For this review, take the finished solid that the model builds, in its own axes (mm). Face numbers are marked on the shaded views. Round coordinates to 2 decimals unless told otherwise and drop trailing zeros. Order: outer loops, then holes, each group sorted by start corner. A loop starts at its lowest first (then second) coordinate and runs counter-clockwise, first axis right, second up.
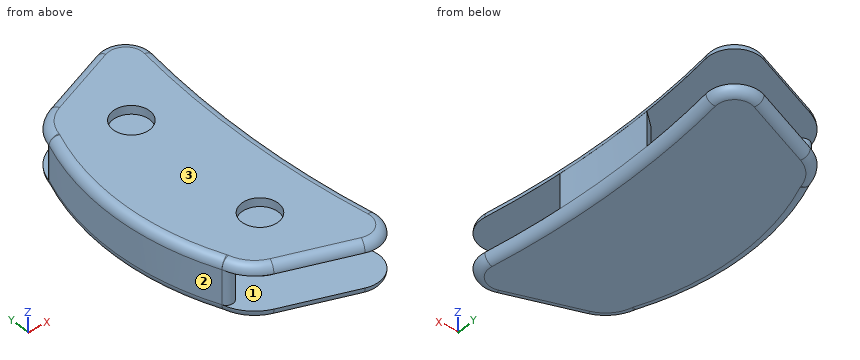
```python
from build123d import *

# Parameters (mm, degrees)
F1_DEPTH  = 2
F2_R      = 5.6
F3_DEPTH  = 1.5
F5_DEPTH  = 10
F7_DEPTH  = 2
F8_R      = 1.99999
F9_R      = 4.25
F10_DEPTH = 2


# Not quite as in the source:
# - a fillet or chamfer is up to 0.001 mm smaller than in the source, because OpenCascade refuses the exact size


with BuildPart() as f1:
    # F0 (on Top) → F1 (new body)
    with BuildSketch(Plane.XY):
        with BuildLine():
            Line((8.2361189543, 36.6168409437), (-7.9935965644, 30.5207371811))
            ThreePointArc((-7.9935965644, 30.5207371811), (-11.9662543406, 27.7862465208), (-14.1970285873, 23.510372898))
            ThreePointArc((-14.1970285873, 23.510372898), (-17, 0), (-14.1970285873, -23.510372898))
            ThreePointArc((-14.1970285873, -23.510372898), (-11.9662543406, -27.7862465208), (-7.9935965644, -30.5207371811))
            Line((-7.9935965644, -30.5207371811), (8.2361189543, -36.6168409437))
            ThreePointArc((8.2361189543, -36.6168409437), (14.1245779615, -35.6606279318), (16.2775548115, -30.0970873786))
            ThreePointArc((16.2775548115, -30.0970873786), (14, 0), (16.2775548115, 30.0970873786))
            ThreePointArc((16.2775548115, 30.0970873786), (14.1245779615, 35.6606279318), (8.2361189543, 36.6168409437))
        make_face()
    extrude(amount=F1_DEPTH)

    # F2 (on face) → F3 (cut)
    with BuildSketch(Plane.XY.offset(2)):
        with Locations((0, 17.5)):
            Circle(F2_R)
        with Locations((0, -17.5)):
            Circle(F2_R)
    extrude(amount=-F3_DEPTH, mode=Mode.SUBTRACT)

    # F4 (on Top) → F5 (join)
    with BuildSketch(Plane.XY):
        with BuildLine():
            Line((-11, -22.8789469535), (-11, 22.8789469535))
            ThreePointArc((-11, 22.8789469535), (-12.3390571638, 24.5083402847), (-14.1970285873, 23.510372898))
            ThreePointArc((-14.1970285873, 23.510372898), (-18.8404213522, 0), (-14.1970285873, -23.510372898))
            ThreePointArc((-14.1970285873, -23.510372898), (-12.3390571638, -24.5083402847), (-11, -22.8789469535))
        make_face()
        with BuildLine():
            Line((14.3490034732, 11.8101475791), (11, 9))
            Line((11, 9), (11, -9))
            Line((11, -9), (14.3490034732, -11.8101475791))
            ThreePointArc((14.3490034732, -11.8101475791), (14, 0), (14.3490034732, 11.8101475791))
        make_face()
    extrude(amount=F5_DEPTH)

    # F6 (on face) → F7 (join)
    with BuildSketch(Plane.XY.offset(10)):
        with BuildLine():
            Line((8.2361189543, 36.6168409437), (-7.9935965644, 30.5207371811))
            ThreePointArc((-7.9935965644, 30.5207371811), (-11.9662543406, 27.7862465208), (-14.1970285873, 23.510372898))
            ThreePointArc((-14.1970285873, 23.510372898), (-12.3390571638, 24.5083402847), (-11, 22.8789469535))
            Line((-11, 22.8789469535), (-11, -22.8789469535))
            ThreePointArc((-11, -22.8789469535), (-12.3390571638, -24.5083402847), (-14.1970285873, -23.510372898))
            ThreePointArc((-14.1970285873, -23.510372898), (-11.9662543406, -27.7862465208), (-7.9935965644, -30.5207371811))
            Line((-7.9935965644, -30.5207371811), (8.2361189543, -36.6168409437))
            ThreePointArc((8.2361189543, -36.6168409437), (14.1245779615, -35.6606279318), (16.2775548115, -30.0970873786))
            ThreePointArc((16.2775548115, -30.0970873786), (14, 0), (16.2775548115, 30.0970873786))
            ThreePointArc((16.2775548115, 30.0970873786), (14.1245779615, 35.6606279318), (8.2361189543, 36.6168409437))
        make_face()
        with BuildLine():
            ThreePointArc((-11, 22.8789469535), (-12.3390571638, 24.5083402847), (-14.1970285873, 23.510372898))
            ThreePointArc((-14.1970285873, 23.510372898), (-18.8404213522, 0), (-14.1970285873, -23.510372898))
            ThreePointArc((-14.1970285873, -23.510372898), (-12.3390571638, -24.5083402847), (-11, -22.8789469535))
            Line((-11, -22.8789469535), (-11, 22.8789469535))
        make_face()
    extrude(amount=F7_DEPTH)

    # F8 (radius 2 in the source; OpenCascade refuses exactly that, so slightly less here)
    f8_edges = [f1.edges().sort_by_distance(p)[0] for p in [
        (14.124578, 35.660628, 12),
        (0.121261, 33.568789, 12),
        (-11.966254, 27.786247, 12),
        (-18.840421, 0, 12),
        (-11.966254, -27.786247, 12),
        (0.121261, -33.568789, 12),
        (14.124578, -35.660628, 12),
        (14, 0, 12),
        (-18.840421, 0, 0),
        (14, 0, 0),
    ]]
    fillet(f8_edges, radius=F8_R)

    # F9 (on face) → F10 (cut)
    with BuildSketch(Plane(origin=(0, 0, 10), x_dir=(1, 0, 0), z_dir=(0, 0, -1))):
        with Locations((0, 17.5)):
            Circle(F9_R)
        with Locations((0, -17.5)):
            Circle(F9_R)
    extrude(amount=-F10_DEPTH, mode=Mode.SUBTRACT)


solid = f1.part
```
Q1. Mouldability with a two-part tool opening along Z and no side actions: class the marked faces 1, 2 and 3 as +Z half, -Z half, draft (parallel to the pull), parting line (faces both ways), or undercut.
Q2. Wall thickness on line 1 (Z direction, x = 12.5, y = 20.5); line 2 (Y direction, x = 0, z = 11); line 3 (X direction, y = 1, z = 9): over which ranges is each line inside the solid? List them lowest first.
Q3. Take a section at A-A, the plane z = 3. State the section outline as (x, y) points, plus the area to 3 significant figures.
Q4. Clearance check with flat-ended pins moving along their axes: pin 1 (6 mm diameter, centred on x = 2.5, y = -11.5, fed in from -Z); pin 2 (4 mm diameter, centred on y = 3.5, z = 5.5, fed in from -X); pin 3 (5 mm diameter, centred on y = -6, z = 4.5, fed in from -X); pin 4 (7.5 mm diameter, centred on x = 0, y = 17.5, fed in from +Z). State where each tip first meets the part, or that it passes through.
Q5. Take a section at B-B, the plane x = 2.5. Count the separate pieces of the cut face and the enclosed holes in it, plus the area to 3 significant figures.
Working result:
1. face 1: undercut
1. face 2: draft
1. face 3: +Z half
2. line 1: z = 0 to 2, 10 to 12
2. line 2: y = -33.24 to -21.75, -13.25 to 13.25, 21.75 to 33.24
2. line 3: x = -18.83 to -11, 11 to 14
3. outline: (-14.2, -23.51) arc R1.66 ccw to (-11, -22.88) - (-11, 22.88) arc R1.66 ccw to (-14.2, 23.51) arc R61.84 ccw to start; (11, -9) - (14.35, -11.81) arc R200 cw to (14.35, 11.81) - (11, 9) - close
3. area: 366 mm2
4. pin 1: stops at z = 0
4. pin 2: stops at x = -18.82
4. pin 3: stops at x = -18.74
4. pin 4: stops at z = 0.5
5. separate pieces: 4
5. enclosed holes: 0
5. area: 214 mm2
